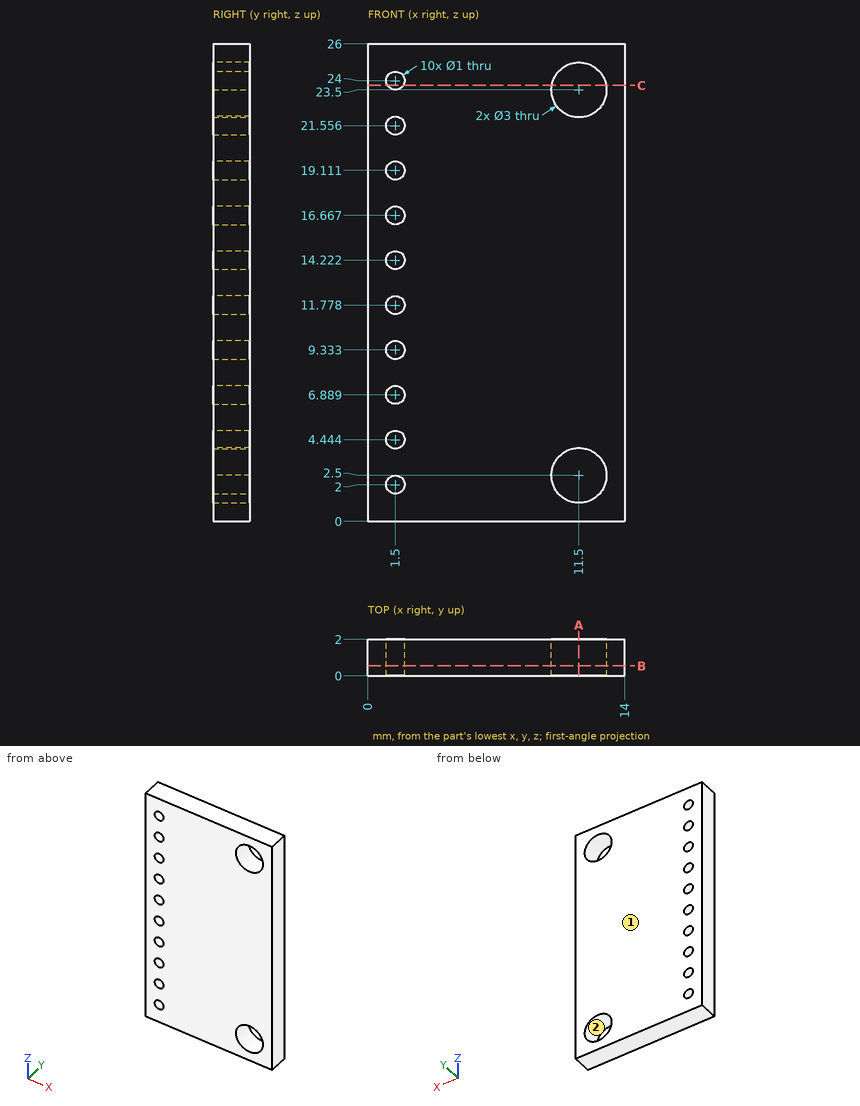
Could you check a few things on this drawing? It's one solid part, dimensions in mm from its lowest x, y, z. Give positions to 0.01 mm unless a question says otherwise; leave off trailing zeros. Write each loop counter-clockwise with the first axis right and the second up, starting at its lowest first coordinate (ties: lowest second). Pieces come first, ordered by that corner, then holes. Notation, with made-up numbers: (15, 27) - (44, 27) arc R21 cw to (44, 64) - close; hole circle Ø1 at (39.25, 77.5). An arc over 180 degrees is marked (long way). Use CSV: the item, a comma, the result in double quotes. Start each with the question number.
Item 1: I want a section at C-C, the plane z = 23.75. Please give me the cut outline in (x, y).
Item 2: If we mould it in two halves opening along Z, with no side actions, what happens to the marked faces 1 and 2? For each: pulls with the +Z half, pulls with the -Z half, needs draft (parallel to the pull), parting line crosses it, or undercut.
Item 3: I'm going to push a flat-ended pin straight in: pin 1 (2.5 mm diameter, centred on x = 11.5, z = 2.5, fed in from -Y). Where does the tip first touch, or does it pass through?
Item 4: I want a section at A-A, the plane x = 11.5. Please give me the cut outline in (y, z), then the cut area to 3 significant figures.
Item 5: If I drill on line 1 along X through (y, z) = (1, 2) (1 decimal); line 2 along X through (y, z) = (0.4, 12); line 3 along Z through (x, y) = (11.25, 1.2), over which ranges is the centre line in solid material (lowest first)?
Item 6: I want a section at B-B, the plane y = 0.55. Give the number of separate pieces and of enclosed holes in the cut face, then the cut area to 3 significant figures.
Findings:
1,outline,"(0, 0) - (1.07, 0) - (1.07, 2) - (0, 2) - close; (1.93, 0) - (10.02, 0) - (10.02, 2) - (1.93, 2) - close; (12.98, 0) - (14, 0) - (14, 2) - (12.98, 2) - close"
2,face 1,"needs draft"
2,face 2,"undercut"
3,pin 1,"passes through"
4,outline,"(0, 0) - (2, 0) - (2, 1) - (0, 1) - close; (0, 4) - (2, 4) - (2, 22) - (0, 22) - close; (0, 25) - (2, 25) - (2, 26) - (0, 26) - close"
4,area,"40.0 mm2"
5,line 1,"x = 0 to 1, 2 to 10.1, 12.9 to 14"
5,line 2,"x = 0 to 1.05, 1.95 to 14"
5,line 3,"z = 0 to 1.02, 3.98 to 22.02, 24.98 to 26"
6,separate pieces,"1"
6,enclosed holes,"12"
6,area,"342 mm2"
